```python
from build123d import *

# Parameters (mm, degrees)
SKETCH1_W           = 10
SKETCH1_H           = 40
BOSS_EXTRUDE1_DEPTH = 7
SKETCH2_R           = 2.125
CUT_EXTRUDE1_DEPTH  = 7
CHAMFER1_SIZE       = 1
SKETCH3_W           = 30
SKETCH3_H           = 7
BOSS_EXTRUDE2_DEPTH = 10
FILLET1_R           = 10


# Some blends are built 0.0001 mm under size
with BuildPart() as part:
    # Sketch1 → Boss-Extrude1 (new body)
    with BuildSketch(Plane.XY):
        with Locations((5, 20)):
            Rectangle(SKETCH1_W, SKETCH1_H)
    extrude(amount=BOSS_EXTRUDE1_DEPTH)

    # Sketch2 → Cut-Extrude1 (cut)
    with BuildSketch(Plane.XY.offset(7)):
        with Locations((5, 35)):
            Circle(SKETCH2_R)
        with Locations((5, 2.5)):
            Circle(SKETCH2_R)
    extrude(amount=-CUT_EXTRUDE1_DEPTH, mode=Mode.SUBTRACT)

    # Chamfer1
    # the kernel refuses this chamfer: 1 mm, written as the material it takes off along each edge
    with BuildSketch(Plane(origin=(5, 35, 7), x_dir=(1, 0, 0), z_dir=(0, -1, 0))) as chamfer1_piece_1:
        Polygon((2.125 + CHAMFER1_SIZE, 0), (2.125, -CHAMFER1_SIZE), (2.125, 0), align=None)
    revolve(axis=Axis((5, 35, 7), (0, 0, 1)), mode=Mode.SUBTRACT)
    with BuildSketch(Plane(origin=(5, 2.5, 7), x_dir=(1, 0, 0), z_dir=(0, -1, 0))) as chamfer1_piece_2:
        Polygon((2.125 + CHAMFER1_SIZE, 0), (2.125, -CHAMFER1_SIZE), (2.125, 0), align=None)
    revolve(axis=Axis((5, 2.5, 7), (0, 0, 1)), mode=Mode.SUBTRACT)

    # Sketch3 → Boss-Extrude2 (add)
    with BuildSketch(Plane.XZ):
        with Locations((5, 3.5)):
            Rectangle(SKETCH3_W, SKETCH3_H)
    extrude(amount=BOSS_EXTRUDE2_DEPTH)

    # Fillet1
    fillet1_edges = [part.edges().sort_by_distance(p)[0] for p in [
        (0, 0, 3.5),
        (10, 0, 3.5),
    ]]
    fillet(fillet1_edges, radius=FILLET1_R - 0.0001)  # a hair under: the kernel refuses the full size


solid = part.part
```
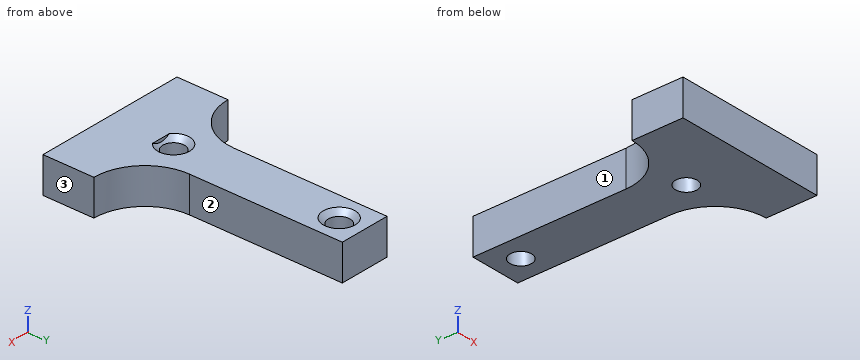
Verification items for the finished model (mm, model axes). Face numbers are marked on the shaded views. A direction names the side the tool comes from. Give positions to 0.01 mm unless a question says otherwise; leave off trailing zeros. Order: outer loops, then holes, each group sorted by start corner. A loop starts at its lowest first (then second) coordinate and runs counter-clockwise, first axis right, second up. Notation, with made-up numbers: M 58.5,33.5 L 94.5,33.5 A30 cw 94.5,69.5 Z; hole C -5.75,80.5 d2. An arc over 180 degrees is marked long. Answer in a Markdown table with one row per item. Add a question column.
Item 1: Section check C-C, the plane z = 1.75. State how many separate pieces and enclosed holes the cut face has, and give its area (3 significant figures).
Item 2: Section check A-A, the plane x = 5. Enter the section's corners in (y, z) (3 decimals), and give its area (3 significant figures).
Item 3: Scan lines: probe 1 along Y at (x, z) = (5, 2.2) (3 decimals); probe 2 along X at (y, z) = (36, 5.75) (3 decimals); probe 3 along X at (y, z) = (29.5, 4). Record each from-to range of solid material in increasing order. Write a range as from..to.
Item 4: Section check D-D, the plane y = 2.5. Enter the section's corners in (x, z) (3 decimals), and give its area (3 significant figures).
Item 5: Gauge pin test, flat ends, axial feed: pin 1 (2 mm diameter, centred on y = 14.5, z = 2.5, fed in from +X); pin 2 (4 mm diameter, centred on x = 5, y = 35, fed in from +Z); pin 3 (2 mm diameter, centred on x = 15.5, z = 5.5, fed in from +Y). Record the tip position at first contact, or that the pin passes through.
Item 6: Section check B-B, the plane y = 35. Enter the section's corners in (x, z) (3 decimals).
Item 7: Tool access check on the marked faces 1, 2 and 3. Record the directions out of +Z, -Z, +X, -X, +Y, -Y that give a thin tool (end or side, any length) a straight path to the whole face; none if there is none.
Filled sheet:
| question | item | result |
|---|---|---|
| 1 | separate pieces | 1 |
| 1 | enclosed holes | 2 |
| 1 | area | 715 mm^2 |
| 2 | outline | M -10,0 L 0.375,0 L 0.375,6 L 0,6.375 L 0,7 L -10,7 Z; M 4.625,0 L 32.875,0 L 32.875,6 L 31.875,7 L 5.625,7 L 4.625,6 Z; M 37.125,0 L 40,0 L 40,7 L 38.125,7 L 37.125,6 Z |
| 2 | area | 289 mm^2 |
| 3 | probe 1 | y = -10..0.375, 4.625..32.875, 37.125..40 |
| 3 | probe 2 | x = 0..3.125, 6.875..10 |
| 3 | probe 3 | x = 0..10 |
| 4 | outline | M -3.386,0 L 2.875,0 L 2.875,6 L 1.875,7 L -3.386,7 Z; M 7.125,0 L 13.386,0 L 13.386,7 L 8.125,7 L 7.125,6 Z |
| 4 | area | 86.6 mm^2 |
| 5 | pin 1 | stops at x = 10 |
| 5 | pin 2 | passes through |
| 5 | pin 3 | stops at y = 1.65 |
| 6 | outline | M 0,0 L 2.875,0 L 2.875,6 L 1.875,7 L 0,7 Z; M 7.125,0 L 10,0 L 10,7 L 8.125,7 L 7.125,6 Z |
| 7 | face 1 | +Z, -Z, -X, +Y |
| 7 | face 2 | +Z, -Z, +X, +Y |
| 7 | face 3 | +Z, -Z, +X, +Y, -Y |
